Autodesk Inventor part; units mm, degrees
ref_plane "YZ Plane" through (0, 0, 0) normal (1, 0, 0) x (0, 1, 0)
ref_plane "XZ Plane" through (0, 0, 0) normal (0, 1, 0) x (-1, 0, 0)
ref_plane "XY Plane" through (0, 0, 0) normal (0, 0, 1) x (1, 0, 0)
sketch "Sketch1" plane through (0, 0, 0) normal (0, 0, 1) x (1, 0, 0)
  line L0 (726.3915, 245.3629) -> (1226.3925, 245.3629)
  line L1 (1476.392, 160.6963) -> (1476.392, 76.0296)
  line L2 (476.392, 76.0296) -> (476.392, 160.6963)
  arc A0 (476.392, 160.6963) -> (726.3915, 245.3629) centre (495.472, 515.784) ccw
  line L3 (1476.392, 118.3629) -> (476.392, 118.3629) construction
  line L4 (976.392, -8.6371) -> (976.392, 245.3629) construction
  arc A1 (726.3915, -8.6371) -> (476.392, 76.0296) centre (495.472, -279.0582) ccw
  arc A2 (1226.3925, 245.3629) -> (1476.392, 160.6963) centre (1457.312, 515.784) ccw
  arc A3 (1476.392, 76.0296) -> (1226.3925, -8.6371) centre (1457.312, -279.0582) ccw
  line L5 (726.3915, -8.6371) -> (1226.3925, -8.6371)
  point P0 (0, 0)
  dimension "d4" = 355.6
  dimension "d5" = 254
  dimension "d6" = 84.6667
extrude "Extrusion1" add sketch "Sketch1" along normal blind 12.7
sketch "Sketch2" plane through (0, 0, 12.7) normal (0, 0, 1) x (1, 0, 0)
  point P0 (0, 0)
move or copy body "Move Body1" bodies to move or copy 1 copy no translate (-1000.125, -123.825, 0)
sketch "Sketch3" plane through (-273.7335, 121.5379, 12.7) normal (0, 0, 1) x (1, 0, 0)
  line L0 (-249.9995, -84.6667) -> (-249.9995, -169.3333) construction
  arc A0 (750.0005, -169.3333) -> (500.001, -254) centre (730.9205, -524.4211) ccw
  line L1 (-249.9995, -84.6667) -> (750.0005, -84.6667) construction
  line L2 (750.0005, -84.6667) -> (750.0005, -169.3333) construction
  line L3 (750.0005, -169.3333) -> (-249.9995, -169.3333) construction
  line L4 (-249.9995, -169.3333) -> (-249.9995, -84.6667) construction
  line L5 (-249.9995, -84.6667) -> (-249.9995, -112.8861) construction
  line L6 (750.0005, -169.3333) -> (750.0005, -84.6667) construction
  line L7 (-249.9995, -112.8861) -> (750.0005, -112.8861) construction
  line L8 (750.0005, -112.8861) -> (750.0005, -141.1055) construction
  line L9 (750.0005, -141.1055) -> (-249.9995, -141.1055) construction
  line L10 (-249.9995, -141.1055) -> (-249.9995, -112.8861) construction
  arc A1 (-249.9995, -84.6667) -> (0, 0) centre (-230.9195, 270.4211) ccw
  line L11 (-211.8394, -84.6667) -> (-211.8394, -169.3333) construction
  arc A2 (0, -254) -> (-249.9995, -169.3333) centre (-230.9195, -524.4211) ccw
  line L12 (-211.8394, -84.6667) -> (-153.2669, -84.6667) construction
  line L13 (-153.2669, -84.6667) -> (-153.2669, -169.3333) construction
  line L14 (-153.2669, -169.3333) -> (-211.8394, -169.3333) construction
  line L15 (-211.8394, -169.3333) -> (-211.8394, -84.6667) construction
  line L16 (500.001, 0) -> (0, 0)
  line L17 (250.0005, 0) -> (250.0005, -254) construction
  point P0 (273.7335, -121.5379)
  point P1 (-211.8394, -112.8861)
  point P2 (-211.8394, -141.1055)
  point P3 (-153.2669, -112.8861)
  point P4 (-153.2669, -141.1055)
  point P5 (711.8404, -112.8861)
  point P6 (711.8404, -141.1055)
  point P7 (653.2679, -112.8861)
  point P8 (653.2679, -141.1055)
  dimension "d15" = 28.2194
  dimension "d16" = 28.2194
hole "Hole1" at (-485.5729, 8.6519, 12.7) at (-427.0004, 8.6519, 12.7) at (-485.5729, -19.5675, 12.7) at (-427.0004, -19.5675, 12.7) at (379.5345, 8.6519, 12.7) at (438.1069, 8.6519, 12.7) at (438.1069, -19.5675, 12.7) at (379.5345, -19.5675, 12.7) direction (0, 0, -1) diameter 6.35 end through all
thread "Thread1"
properties part number "Electric Skateboard Deck"
The listing builds one solid part. Answer for the finished solid, in the listing's coordinates (mm). Give positions to 0.01 mm unless a question says otherwise; leave off trailing zeros. Order: outer loops, then holes, each group sorted by start corner. A loop starts at its lowest first (then second) coordinate and runs counter-clockwise, first axis right, second up. Notation, with made-up numbers: (43.25, 32) - (49.25, 32) arc R30 cw to (49.25, 54) - close; hole circle Ø1 at (12, -25). An arc over 180 degrees is marked (long way). One line per item, written item: value. Start each with the question number.
1) A cutting plane is placed at B-B on y = -106.5. Give the vertices of the cut face in (x, z).
2) Find the intervals of material crossed by L1, parallel to X at y = -20.5, z = 10.25; L2, parallel to Y at x = 381.5, z = 1.75; L3, parallel to Y at x = 377, z = 11.5, in increasing order.
3) A cutting plane is placed at A-A on z = 2. State how many separate pieces and enclosed holes the cut face has, then the cut area to 3 significant figures.
4) The mould has two halves that part along Y. Classify faces 1 (the face through (-392.381, -65.472, 6.261)), 2 (the face through (-388.8, 55.76, 6.26)), 3 (the face through (-31, -4, 0)): released by +Y, released by -Y, zero draft, split by the parting line, or undercut.
5) Given pin 1 Ø5.5 at (x, y) = (-427, 8.65) entering from -Z; pin 2 Ø5 at (x, z) = (-364, 3.5) entering from +Y; pin 3 Ø4 at (y, z) = (-89, 2) entering from -X, each flat-ended and moving along its own axis, determine where each tip first touches the part or whether it passes through.
6) A cutting plane is placed at C-C on x = 317.5. Give the vertices of the cut face in (y, z), then the cut area to 3 significant figures.
Answer sheet:
1. outline: (-308.16, 0) - (260.7, 0) - (260.7, 12.7) - (-308.16, 12.7) - close
2. L1: x = -523.73 to -488.61, -482.54 to -430.04, -423.97 to 376.5, 382.57 to 435.07, 441.14 to 476.27
2. L2: y = -55.43 to -22.06, -17.07 to 6.16, 11.15 to 44.51
2. L3: y = -56.44 to -21.48, -17.66 to 6.74, 10.56 to 45.52
3. separate pieces: 1
3. enclosed holes: 8
3. area: 193,000 mm2
4. face 1: released by -Y
4. face 2: released by +Y
4. face 3: zero draft
5. pin 1: passes through
5. pin 2: stops at y = 66.45
5. pin 3: stops at x = -341.35
6. outline: (-75.87, 0) - (64.94, 0) - (64.94, 12.7) - (-75.87, 12.7) - close
6. area: 1,790 mm2
